Geometry check sheet. Reference: the model listing, model coordinates, mm. A direction names the side the tool comes from. Give positions to 0.01 mm unless a question says otherwise; leave off trailing zeros. Loops run counter-clockwise (first coordinate to the right, second up) from the corner with the lowest first, then second, coordinate; pieces in that order, holes last.
1. Go/stop test with flat-tipped pins: pin 1 Ø2.5 at (x, y) = (0.5, -2) entering from +Z; pin 2 Ø8 at (x, y) = (19.5, 15) entering from -Z; pin 3 Ø3 at (x, z) = (4.5, -48.5) entering from +Y. Record where each tip stops, or that it passes through.
2. Tool access check on faces 5 (the cylindrical face through (2.855, -6.363, -39.74)), 6 (the flat face through (-16, 16, 0)), 7 (the cylindrical face through (-12.013, -22.753, -15.21)), 8 (the cylindrical face through (23.121, -16.183, -15.21)), 9 (the flat face through (20, 16, -30)). Record the directions out of +Z, -Z, +X, -X, +Y, -Y that give a thin tool (end or side, any length) a straight path to the whole face; none if there is none.
3. Release check for a two-part mould opening along Y. For faces 1 (the flat face through (19.985, 15.738, -14.79)), 2 (the flat face through (-1, -13, -38.7)), 3 (the cylindrical face through (-14.668, -17.547, -36.465)), 4 (the cylindrical face through (16.572, -22.745, -15.21)) record: +Y half, -Y half, draft (parallel to the pull), parting line (faces both ways), or undercut.
4. Cross-section at C-C, the plane z = -37.5. Record the cut outline in (x, y), plus the area to 3 significant figures.
5. Cross-section at D-D, the plane y = 10. Record the cut outline in (x, z), plus the area to 3 significant figures.
6. Cross-section at B-B, the plane y = 16. Record the cut outline in (x, z), plus the area to 3 significant figures.
7. Cross-section at A-A, the plane z = -13. Record the cut outline in (x, y).
8. Material ranges on L1, parallel to Z at x = 4.5, y = 12; L2, parallel to Z at x = 9, y = 6.5; L3, parallel to Y at x = 1, z = -39.5, recorded low to high.
Autodesk Inventor part; units mm, degrees
ref_plane "YZ Plane" through (0, 0, 0) normal (1, 0, 0) x (0, 1, 0)
ref_plane "XZ Plane" through (0, 0, 0) normal (0, 1, 0) x (-1, 0, 0)
ref_plane "XY Plane" through (0, 0, 0) normal (0, 0, 1) x (1, 0, 0)
sketch "Szkic1" plane through (0, 0, 0) normal (0, 0, 1) x (1, 0, 0)
  line L0 (-18.7306, 19.0987) -> (23.2694, 19.0987)
  line L1 (23.2694, 19.0987) -> (23.2694, -22.9013)
  line L2 (23.2694, -22.9013) -> (-18.7306, -22.9013)
  line L3 (-18.7306, -22.9013) -> (-18.7306, 19.0987)
  point P0 (0, 0)
  dimension "d0" = 42
  dimension "d1" = 42
extrude "Wyciągnięcie proste1" add sketch "Szkic1" along normal blind 9
chamfer "Faza1" distance 2 angle 45 4 edges at (23.2694, 19.0987, 4.5) (-18.7306, 19.0987, 4.5) (-18.7306, -22.9013, 4.5) (23.2694, -22.9013, 4.5)
sketch "Szkic2" plane through (0, 0, 0) normal (0, 0, -1) x (-1, 0, 0)
  line L0 (-21.2694, -22.9013) -> (-23.2694, -20.9013)
  line L1 (-21.2694, -22.9013) -> (16.7306, -22.9013)
  line L2 (18.7306, -20.9013) -> (16.7306, -22.9013)
  line L3 (18.7306, -20.9013) -> (18.7306, 17.0987)
  line L4 (16.7306, 19.0987) -> (18.7306, 17.0987)
  line L5 (16.7306, 19.0987) -> (-21.2694, 19.0987)
  line L6 (-23.2694, 17.0987) -> (-21.2694, 19.0987)
  line L7 (-23.2694, 17.0987) -> (-23.2694, -20.9013)
  line L8 (12.0859, 19.0987) -> (-16.6247, 19.0987)
  line L9 (-23.2694, -16.2567) -> (-16.6247, -22.9013)
  line L10 (12.0859, -22.9013) -> (18.7306, -16.2567)
  line L11 (-23.2694, 12.454) -> (-16.6247, 19.0987)
  line L12 (12.0859, 19.0987) -> (18.7306, 12.454)
  line L13 (-16.6247, 19.0987) -> (12.0859, 19.0987)
  line L14 (-23.2694, 17.0987) -> (-23.2694, -20.9013)
  line L15 (-23.2694, 12.454) -> (-23.2694, -16.2567)
  line L16 (-23.2694, -16.2567) -> (-23.2694, 12.454)
  line L17 (-16.6247, -22.9013) -> (12.0859, -22.9013)
  line L18 (-16.6247, -22.9013) -> (12.0859, -22.9013)
  line L19 (18.7306, -16.2567) -> (18.7306, 12.454)
  point P0 (0, 0)
  point P1 (-2.2694, -1.9013)
  dimension "d9" = 21
  dimension "d10" = 42
  dimension "d11" = 21
  dimension "d12" = 25
  dimension "d13" = 25
  dimension "d14" = 25
  dimension "d15" = 25
extrude "Wyciągnięcie proste3" add sketch "Szkic2" along normal blind 30 contours L9 L7 L11 L5 L12 L3 L10 L1
sketch "Szkic3" plane through (0, 0, -30) normal (0, 0, -1) x (-1, 0, 0)
  line L0 (-23.2694, -16.2567) -> (-16.6247, -22.9013)
  line L1 (-16.6247, -22.9013) -> (12.0859, -22.9013)
  line L2 (12.0859, -22.9013) -> (18.7306, -16.2567)
  line L3 (18.7306, -16.2567) -> (18.7306, 12.454)
  line L4 (18.7306, 12.454) -> (12.0859, 19.0987)
  line L5 (12.0859, 19.0987) -> (-16.6247, 19.0987)
  line L6 (-16.6247, 19.0987) -> (-23.2694, 12.454)
  line L7 (-23.2694, 12.454) -> (-23.2694, -16.2567)
  line L8 (-23.2694, 12.454) -> (-16.6247, 19.0987)
  line L9 (-16.6247, 19.0987) -> (-21.2694, 19.0987)
  line L10 (-23.2694, 17.0987) -> (-21.2694, 19.0987)
  line L11 (-23.2694, 17.0987) -> (-23.2694, 12.454)
  line L12 (-16.6247, -22.9013) -> (-23.2694, -16.2567)
  line L13 (-23.2694, -16.2567) -> (-23.2694, -20.9013)
  line L14 (-21.2694, -22.9013) -> (-23.2694, -20.9013)
  line L15 (-21.2694, -22.9013) -> (-16.6247, -22.9013)
  line L16 (18.7306, -16.2567) -> (12.0859, -22.9013)
  line L17 (12.0859, -22.9013) -> (16.7306, -22.9013)
  line L18 (18.7306, -20.9013) -> (16.7306, -22.9013)
  line L19 (18.7306, -20.9013) -> (18.7306, -16.2567)
  line L20 (12.0859, 19.0987) -> (18.7306, 12.454)
  line L21 (18.7306, 12.454) -> (18.7306, 17.0987)
  line L22 (16.7306, 19.0987) -> (18.7306, 17.0987)
  line L23 (16.7306, 19.0987) -> (12.0859, 19.0987)
  line L24 (-23.2694, 19.0987) -> (-23.2694, -22.9013)
  line L25 (-23.2694, -22.9013) -> (18.7306, -22.9013)
  line L26 (18.7306, -22.9013) -> (18.7306, 19.0987)
  line L27 (18.7306, 19.0987) -> (-23.2694, 19.0987)
  point P0 (0, 0)
extrude "Wyciągnięcie proste4" add sketch "Szkic3" along normal blind 9 contours L7 L6 L5 L4 L3 L2 L1 L0 | L0 L15 L14 L13 | L11 L10 L9 L6 | L2 L19 L18 L17 | L23 L22 L21 L4
fillet "Zaokrąglenie1" radius 2 8 edges at (-18.7306, 12.454, -15) (-12.0859, 19.0987, -15) (16.6247, 19.0987, -15) (23.2694, 12.454, -15) (-18.7306, -16.2567, -15) (-12.0859, -22.9013, -15) (16.6247, -22.9013, -15) (23.2694, -16.2567, -15)
sketch "Szkic4" plane through (0, 0, 9) normal (0, 0, 1) x (1, 0, 0)
  line L0 (-18.7306, 17.0987) -> (-18.7306, -20.9013)
  line L1 (23.2694, -20.9013) -> (23.2694, 17.0987)
  line L2 (21.2694, 19.0987) -> (-16.7306, 19.0987)
  circle A0 centre (2.2694, -1.9013) radius 4.5
  line L3 (23.2694, 19.0987) -> (-18.7306, 19.0987)
  line L4 (23.2694, -22.9013) -> (-18.7306, -22.9013)
  line L5 (21.2694, -22.9013) -> (-16.7306, -22.9013)
  line L6 (-18.7306, -22.9013) -> (-18.7306, 19.0987)
  line L7 (23.2694, 19.0987) -> (23.2694, -22.9013)
  point P0 (0, 0)
  dimension "d21" = 42
  dimension "d22" = 21
  dimension "d23" = 21
  dimension "d24" = 9
extrude "Wyciągnięcie proste5" cut sketch "Szkic4" against normal blind 4 contours A0
fillet "Zaokrąglenie2" radius 0.6 16 edges at (23.2694, -1.9013, 9) (2.2694, -22.9013, 9) (-18.7306, -1.9013, 9) (2.2694, 19.0987, 9) (22.2694, -21.9013, 9) (-17.7306, -21.9013, 9) (-17.7306, 18.0987, 9) (22.2694, 18.0987, 9) (23.2694, -1.9013, -39) (22.2694, 18.0987, -39) (2.2694, 19.0987, -39) (-17.7306, 18.0987, -39) (-18.7306, -1.9013, -39) (-17.7306, -21.9013, -39) (2.2694, -22.9013, -39) (22.2694, -21.9013, -39)
sketch "Szkic5" plane through (0, 0, -39) normal (0, 0, -1) x (-1, 0, 0)
  circle A0 centre (-2.2694, -1.9013) radius 4.5
  line L0 (-21.2694, -22.9013) -> (16.7306, -22.9013)
  line L1 (16.7306, -22.9013) -> (18.7306, -20.9013)
  line L2 (18.7306, -20.9013) -> (18.7306, 17.0987)
  line L3 (18.7306, 17.0987) -> (16.7306, 19.0987)
  line L4 (16.7306, 19.0987) -> (-21.2694, 19.0987)
  line L5 (-21.2694, 19.0987) -> (-23.2694, 17.0987)
  line L6 (-23.2694, 17.0987) -> (-23.2694, -20.9013)
  line L7 (-23.2694, -20.9013) -> (-21.2694, -22.9013)
  line L8 (18.7306, -22.9013) -> (18.7306, 19.0987)
  line L9 (18.7306, 19.0987) -> (-23.2694, 19.0987)
  line L10 (-23.2694, 19.0987) -> (-23.2694, -22.9013)
  line L11 (-23.2694, -22.9013) -> (18.7306, -22.9013)
  circle A1 centre (-2.2694, -1.9013) radius 11
  circle A2 centre (-2.2694, -1.9013) radius 16.25
  circle A3 centre (-2.2694, -1.9013) radius 2.5
  point P0 (0, 0)
  point P1 (13.1806, -17.3513)
  point P2 (13.1806, 13.5487)
  point P3 (-17.7194, 13.5487)
  point P4 (-17.7194, -17.3513)
  dimension "d28" = 42
  dimension "d29" = 5.55
  dimension "d30" = 5.55
  dimension "d31" = 5.55
  dimension "d32" = 5.55
  dimension "d33" = 5.55
  dimension "d34" = 5.55
  dimension "d35" = 5.55
  dimension "d36" = 5.55
  dimension "d37" = 22
  dimension "d38" = 32.5
  dimension "d53" = 5
extrude "Wyciągnięcie proste6" cut sketch "Szkic5" against normal blind 0.3 contours A2
extrude "Wyciągnięcie proste7" add sketch "Szkic5" along normal blind 2 contours A1
chamfer "Faza2" distance 0.5 angle 45 1 edges at (6.7694, -1.9013, -41)
hole "Otwór1" at (-13.1806, -17.3513, -39) at (-13.1806, 13.5487, -39) at (17.7194, 13.5487, -39) at (17.7194, -17.3513, -39) direction (0, 0, 1) diameter 3 depth 5 tip angle 118
extrude "Wyciągnięcie proste8" add sketch "Szkic5" along normal blind 25 contours A3
properties part number "COTS_GENERIC_NEMA17_25mm_shaft"
Result:
1. pin 1: stops at z = 5
1. pin 2: stops at z = -39
1. pin 3: stops at y = 0.49
2. face 5: -Z
2. face 6: -X, +Y
2. face 7: -X, -Y
2. face 8: +X, -Y
2. face 9: +X, +Y
3. face 1: +Y half
3. face 2: undercut
3. face 3: undercut
3. face 4: -Y half
4. outline: (-18.73, -20.9) - (-16.73, -22.9) - (21.27, -22.9) - (23.27, -20.9) - (23.27, 17.1) - (21.27, 19.1) - (-16.73, 19.1) - (-18.73, 17.1) - close; hole circle Ø3 at (-13.18, -17.35); hole circle Ø3 at (-13.18, 13.55); hole circle Ø3 at (17.72, -17.35); hole circle Ø3 at (17.72, 13.55)
4. area: 1,730 mm2
5. outline: (-18.73, -38.4) arc R0.6 ccw to (-18.13, -39) - (-8.8, -39) - (-8.8, -38.7) - (13.33, -38.7) - (13.33, -39) - (22.67, -39) arc R0.6 ccw to (23.27, -38.4) - (23.27, 8.4) arc R0.6 ccw to (22.67, 9) - (-18.13, 9) arc R0.6 ccw to (-18.73, 8.4) - close
5. area: 2,010 mm2
6. outline: (-18.73, -38.4) arc R0.6 ccw to (-18.13, -39) - (22.67, -39) arc R0.6 ccw to (23.27, -38.4) - (23.27, -30) - (19.72, -30) - (19.72, 0) - (23.27, 0) - (23.27, 8.4) arc R0.6 ccw to (22.67, 9) - (-18.13, 9) arc R0.6 ccw to (-18.73, 8.4) - (-18.73, 0) - (-15.18, 0) - (-15.18, -30) - (-18.73, -30) - close
6. area: 1,800 mm2
7. outline: (-18.73, -15.43) arc R2 ccw to (-18.14, -16.84) - (-12.67, -22.32) arc R2 ccw to (-11.26, -22.9) - (15.8, -22.9) arc R2 ccw to (17.21, -22.32) - (22.68, -16.84) arc R2 ccw to (23.27, -15.43) - (23.27, 11.63) arc R2 ccw to (22.68, 13.04) - (17.21, 18.51) arc R2 ccw to (15.8, 19.1) - (-11.26, 19.1) arc R2 ccw to (-12.67, 18.51) - (-18.14, 13.04) arc R2 ccw to (-18.73, 11.63) - close
8. L1: z = -38.7 to 9
8. L2: z = -41 to 9
8. L3: y = -12.83 to -6.22, -4.06 to 0.25, 2.42 to 9.03
